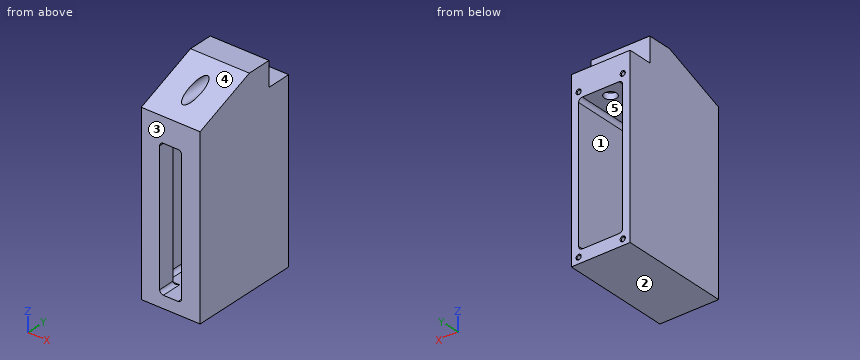
from build123d import *

# Parameters (mm, degrees)
BOSS_EXTRUDE1_DEPTH            = 9
BOSS_EXTRUDE2_DEPTH            = 6
SKETCH3_W                      = 10
SKETCH3_H                      = 90
BOSS_EXTRUDE3_DEPTH            = 9
FILLET1_R                      = 3
FILLET1_OF_MIRROR4_R           = 3
FILLET2_R                      = 3
F_2_5MM_DOWEL_HOLE1_D          = 3.2
F_2_5MM_DOWEL_HOLE1_DEPTH      = 6.5
F_2_5MM_DOWEL_HOLE1_TIP        = 0.96137699
CHAMFER1_SIZE                  = 0.5
SKETCH8_R                      = 5
CUT_EXTRUDE1_DEPTH             = 158.203689524
CBORE_FOR_M5_SHCS2_D           = 5.5
CBORE_FOR_M5_SHCS2_DEPTH       = 40
CBORE_FOR_M5_SHCS2_CBORE_D     = 10
CBORE_FOR_M5_SHCS2_CBORE_DEPTH = 5


with BuildPart() as part:
    # Sketch1 → Boss-Extrude1 (new body)
    with BuildSketch(Plane(origin=(0, 0, 0), x_dir=(0, 0, -1), z_dir=(1, 0, 0))):
        Polygon((0, 0), (0, -20), (-20, -20), (-20, -40), (0, -90), (143, -90), (143, 0), (133, 0), (133, -76.5), (20, -76.5), (20, 0), align=None)
    boss_extrude1 = extrude(amount=BOSS_EXTRUDE1_DEPTH)

    # Sketch2 → Boss-Extrude2 (add)
    with BuildSketch(Plane.ZY):
        Polygon((0, 0), (-143, 0), (-143, -90), (0, -90), (20, -40), (20, -20), (0, -20), align=None)
    boss_extrude2 = extrude(amount=BOSS_EXTRUDE2_DEPTH)

    # Sketch3 → Boss-Extrude3 (add)
    with BuildSketch(Plane(origin=(9, 0, 0), x_dir=(0, 0, -1), z_dir=(1, 0, 0))):
        Polygon((0, -90), (20, -90), (20, 0), (0, 0), (0, -20), (-20, -20), (-20, -40), align=None)
        with Locations((138, -45)):
            Rectangle(SKETCH3_W, SKETCH3_H)
    boss_extrude3 = extrude(amount=BOSS_EXTRUDE3_DEPTH)

    # Fillet1
    fillet1_edges = [part.edges().sort_by_distance(p)[0] for p in [
        (4.5, -76.5, -20),
        (4.5, -76.5, -133),
        (9, -83.25, -133),
        (9, -83.25, -20),
    ]]
    fillet(fillet1_edges, radius=FILLET1_R)

    # Mirror4: Boss-Extrude1, Boss-Extrude2, Boss-Extrude3 across plane
    add(boss_extrude1.mirror(Plane(origin=(18, 0, 0), x_dir=(0, 0, 1), z_dir=(1, 0, 0))))
    add(boss_extrude2.mirror(Plane(origin=(18, 0, 0), x_dir=(0, 0, 1), z_dir=(1, 0, 0))))
    add(boss_extrude3.mirror(Plane(origin=(18, 0, 0), x_dir=(0, 0, 1), z_dir=(1, 0, 0))))

    # Fillet1 of Mirror4
    fillet1_of_mirror4_edges = [part.edges().sort_by_distance(p)[0] for p in [
        (31.5, -76.5, -20),
        (31.5, -76.5, -133),
        (27, -83.25, -133),
        (27, -83.25, -20),
    ]]
    fillet(fillet1_of_mirror4_edges, radius=FILLET1_OF_MIRROR4_R)

    # Fillet2
    fillet2_edges = [part.edges().sort_by_distance(p)[0] for p in [
        (36, -76.5, -76.5),
        (36, -36.75, -20),
        (36, -36.75, -133),
        (36, -75.621320344, -20.878679656),
        (36, -75.621320344, -132.121320344),
        (0, -36.75, -133),
        (0, -36.75, -20),
        (0, -76.5, -76.5),
        (0, -75.621320344, -20.878679656),
        (0, -75.621320344, -132.121320344),
    ]]
    fillet(fillet2_edges, radius=FILLET2_R)

    # Ø2.5mm Dowel Hole1
    with Locations(Plane(origin=(0, 0, 0), x_dir=(1, 0, 0), z_dir=(0, 1, 0))):
        with Locations((36, 138), (0, 138), (0, 15), (36, 15)):
            Hole(F_2_5MM_DOWEL_HOLE1_D / 2, depth=F_2_5MM_DOWEL_HOLE1_DEPTH)
            with Locations((0, 0, -(F_2_5MM_DOWEL_HOLE1_DEPTH + F_2_5MM_DOWEL_HOLE1_TIP / 2))):  # 118° drill point
                Cone(0, F_2_5MM_DOWEL_HOLE1_D / 2, F_2_5MM_DOWEL_HOLE1_TIP, mode=Mode.SUBTRACT)

    # Chamfer1
    chamfer1_edges = [part.edges().sort_by_distance(p)[0] for p in [
        (37.6, 0, -138),
        (37.6, 0, -15),
        (1.6, 0, -15),
        (1.6, 0, -138),
    ]]
    chamfer(chamfer1_edges, length=CHAMFER1_SIZE)

    # Sketch7 → CBORE for M5 SHCS1 (revolve, cut)
    with BuildSketch(Plane(origin=(18, -40, 10), x_dir=(0, 0, -1), z_dir=(1, 0, 0))):
        Polygon((0, 0), (0, 40), (2.75, 40), (2.75, 5), (5, 5), (5, 0), align=None)
    revolve(axis=Axis((18, -46.35, 10), (0, 1, 0)), mode=Mode.SUBTRACT)

    # Sketch8 → Cut-Extrude1 (cut, through all)
    with BuildSketch(Plane(origin=(0, -40, 0), x_dir=(1, 0, 0), z_dir=(0, 1, 0))):
        with Locations(Location((18, -10, 0), (0, 0, 90))):
            Circle(SKETCH8_R)
    extrude(amount=-CUT_EXTRUDE1_DEPTH, mode=Mode.SUBTRACT)

    # CBORE for M5 SHCS2
    with Locations(Plane(origin=(0, 0, -20), x_dir=(-1, 0, 0), z_dir=(0, 0, -1))):
        with Locations((-18, -10)):
            CounterBoreHole(CBORE_FOR_M5_SHCS2_D / 2, CBORE_FOR_M5_SHCS2_CBORE_D / 2, CBORE_FOR_M5_SHCS2_CBORE_DEPTH, depth=CBORE_FOR_M5_SHCS2_DEPTH)


solid = part.part
Geometry: final body of the model. Coordinates: model frame, mm. Face numbers are marked on the shaded views. A direction names the side the tool comes from. Give positions to 0.01 mm unless a question says otherwise; leave off trailing zeros. Write each loop counter-clockwise with the first axis right and the second up, starting at its lowest first coordinate (ties: lowest second). Pieces come first, ordered by that corner, then holes. Notation, with made-up numbers: (86, -2.5) -> (105, -2.5) arc R18 ccw to (105, 26.5) -> close; hole circle Ø4 at (-24.5, -13.5). An arc over 180 degrees is marked (long way). Answer in a Markdown table with one row per item.
(1) Set-up query: the marked faces 4 and 5. Return all of +Z, -Z, +X, -X, +Y, -Y with unobstructed straight access to the full face (end or side cutting, diameter ignored); none if empty.
Answers below:
| item | result |
|---|---|
| face 4 | +Z, +X, -X, -Y |
| face 5 | +Y |
(2) Section query B-B on x = 18. Return loops of the section in (y, z), then the cut area to 4 significant figures.
Answers below:
| item | result |
|---|---|
| outline | (-90, -143) -> (0, -143) -> (0, -133) -> (-90, -133) -> close; (-90, -20) -> (-15, -20) -> (-15, -15) -> (-12.75, -15) -> (-12.75, 0) -> (-20, 0) -> (-20, 7.25) -> (-35, 7.25) -> (-35, 5) -> (-77.5, 5) -> (-90, 0) -> close; (-52.5, 15) -> (-35, 15) -> (-35, 12.75) -> (-20, 12.75) -> (-20, 20) -> (-40, 20) -> close; (-7.25, -15) -> (-5, -15) -> (-5, -20) -> (0, -20) -> (0, 0) -> (-7.25, 0) -> close |
| area | 3,085 mm^2 |
(3) Section query D-D on y = -61.5. Return loops of the section in (x, z).
Answers below:
| item | result |
|---|---|
| outline | (-6, -143) -> (42, -143) -> (42, 11.4) -> (22.8, 11.4) arc R5 cw (long way) to (13.2, 11.4) -> (-6, 11.4) -> close; hole (0, -130) arc R3 ccw to (3, -133) -> (33, -133) arc R3 ccw to (36, -130) -> (36, -23) arc R3 ccw to (33, -20) -> (3, -20) arc R3 ccw to (0, -23) -> close |
(4) Section query A-A on y = -52. Return loops of the section in (x, z), then the cut area to 3 significant figures.
Answers below:
| item | result |
|---|---|
| outline | (-6, -143) -> (42, -143) -> (42, 15.2) -> (-6, 15.2) -> close; hole (0, -130) arc R3 ccw to (3, -133) -> (33, -133) arc R3 ccw to (36, -130) -> (36, -23) arc R3 ccw to (33, -20) -> (3, -20) arc R3 ccw to (0, -23) -> close; hole circle Ø10 at (18, 10) |
| area | 3,450 mm^2 |
(5) Ray query, line 1 along Z through (x, y) = (18, -30.75); line 2 along X through (y, z) = (-1.7, -15); line 3 along Z through (x, y) = (18, -37.75). Return the intervals inside material, ascending. Write a range as [from, to].
Answers below:
| item | result |
|---|---|
| line 1 | [-143, -133], [-20, 7.25], [12.75, 20] |
| line 2 | [-6, -1.6], [1.6, 34.4], [37.6, 42] |
| line 3 | [-143, -133], [-20, 5], [15, 20] |
(6) Draft query along Z for the marked faces 1, 2 and 3. Return one class per face: +Z half, -Z half, draft (parallel to the pull), parting line (faces both ways), or undercut.
Answers below:
| item | result |
|---|---|
| face 1 | undercut |
| face 2 | -Z half |
| face 3 | draft |
(7) Pin query (flat end, axial travel): pin 1 (1.8 mm diameter, centred on x = 29, z = -50.5, fed in from +Y); pin 2 (8 mm diameter, centred on x = 18, y = -10, fed in from +Z); pin 3 (22 mm diameter, centred on x = 28, y = -13.5, fed in from +Z); pin 4 (5 mm diameter, centred on x = 18, z = 10, fed in from +Y). Return the tip coordinate at first contact, or that it passes through.
Answers below:
| item | result |
|---|---|
| pin 1 | y = -76.5 |
| pin 2 | z = 0 |
| pin 3 | z = 20 |
| pin 4 | through |
(8) Section query C-C on z = -75.5. Return loops of the section in (x, y), then the cut area to 3 significant figures.
Answers below:
| item | result |
|---|---|
| outline | (-6, -90) -> (9, -90) -> (9, -76.5) -> (3, -76.5) arc R3 cw to (0, -73.5) -> (0, 0) -> (-6, 0) -> close; (27, -90) -> (42, -90) -> (42, 0) -> (36, 0) -> (36, -73.5) arc R3 cw to (33, -76.5) -> (27, -76.5) -> close |
| area | 1,330 mm^2 |
